Verification items for the finished model (mm, model axes). Round coordinates to 2 decimals unless told otherwise and drop trailing zeros. Write each loop counter-clockwise with the first axis right and the second up, starting at its lowest first coordinate (ties: lowest second). Pieces come first, ordered by that corner, then holes.
from build123d import *

# Parameters (mm, degrees)
GENERICCARDPCBDEFINITION_FILLET3_START   = -0.8
GENERICCARDPCBDEFINITION_FILLET3_OUTLI_R = 0.16
GENERICCARDPCBDEFINITION_FILLET3_DEPTH   = 1.6
SKETCH1_R                                = 1.1
CUT_EXTRUDE1_DEPTH                       = 10


# Read off the part's stored shape, not the designer's step: <GenericCardPCBDefinition>-<Fillet3>
with BuildPart() as part:
    # <GenericCardPCBDefinition>-<Fillet3> outli → <GenericCardPCBDefinition>-<Fillet3> (new body)
    with BuildSketch(Plane(origin=(0, 0, 0), x_dir=(1, 0, 0), z_dir=(0, 1, 0)).offset(GENERICCARDPCBDEFINITION_FILLET3_START)):
        with BuildLine():
            ThreePointArc((-41.232050808, -44.8), (-40.5, -44.067949192), (-39.5, -43.8))
            Line((-39.5, -43.8), (-38.267949192, -43.8))
            ThreePointArc((-38.267949192, -43.8), (-37.914395801, -43.653553391), (-37.767949192, -43.3))
            Line((-37.767949192, -43.3), (-37.767949192, -41.3))
            ThreePointArc((-37.767949192, -41.3), (-37.621502583, -40.946446609), (-37.267949192, -40.8))
            Line((-37.267949192, -40.8), (-35.59, -40.8))
            Line((-35.59, -40.8), (-35.59, -37.1))
            ThreePointArc((-35.59, -37.1), (-35.443553391, -36.746446609), (-35.09, -36.6))
            Line((-35.09, -36.6), (-32.91, -36.6))
            ThreePointArc((-32.91, -36.6), (-32.556446609, -36.746446609), (-32.41, -37.1))
            Line((-32.41, -37.1), (-32.41, -40.8))
            Line((-32.41, -40.8), (-29.59, -40.8))
            Line((-29.59, -40.8), (-29.59, -37.1))
            ThreePointArc((-29.59, -37.1), (-29.443553391, -36.746446609), (-29.09, -36.6))
            Line((-29.09, -36.6), (-26.91, -36.6))
            ThreePointArc((-26.91, -36.6), (-26.556446609, -36.746446609), (-26.41, -37.1))
            Line((-26.41, -37.1), (-26.41, -40.8))
            Line((-26.41, -40.8), (-23.59, -40.8))
            Line((-23.59, -40.8), (-23.59, -37.1))
            ThreePointArc((-23.59, -37.1), (-23.443553391, -36.746446609), (-23.09, -36.6))
            Line((-23.09, -36.6), (-20.91, -36.6))
            ThreePointArc((-20.91, -36.6), (-20.556446609, -36.746446609), (-20.41, -37.1))
            Line((-20.41, -37.1), (-20.41, -40.8))
            Line((-20.41, -40.8), (-18.732050808, -40.8))
            ThreePointArc((-18.732050808, -40.8), (-18.378497417, -40.946446609), (-18.232050808, -41.3))
            Line((-18.232050808, -41.3), (-18.232050808, -43.3))
            ThreePointArc((-18.232050808, -43.3), (-18.085604199, -43.653553391), (-17.732050808, -43.8))
            Line((-17.732050808, -43.8), (-16.5, -43.8))
            ThreePointArc((-16.5, -43.8), (-15.5, -44.067949192), (-14.767949192, -44.8))
            Line((-14.767949192, -44.8), (14.767949192, -44.8))
            ThreePointArc((14.767949192, -44.8), (16.5, -43.8), (18.232050808, -44.8))
            Line((18.232050808, -44.8), (37.767949192, -44.8))
            ThreePointArc((37.767949192, -44.8), (39.5, -43.8), (41.232050808, -44.8))
            Line((41.232050808, -44.8), (44.1, -44.8))
            Line((44.1, -44.8), (49.9, -39))
            Line((49.9, -39), (49.9, 40.9))
            ThreePointArc((49.9, 40.9), (49.753553391, 41.253553391), (49.4, 41.4))
            Line((49.4, 41.4), (47.65, 41.4))
            ThreePointArc((47.65, 41.4), (47.296446609, 41.546446609), (47.15, 41.9))
            Line((47.15, 41.9), (47.15, 45.8))
            ThreePointArc((47.15, 45.8), (47.003553391, 46.153553391), (46.65, 46.3))
            Line((46.65, 46.3), (34.9, 46.3))
            ThreePointArc((34.9, 46.3), (34.546446609, 46.446446609), (34.4, 46.8))
            Line((34.4, 46.8), (34.4, 49.4))
            ThreePointArc((34.4, 49.4), (34.253553391, 49.753553391), (33.9, 49.9))
            Line((33.9, 49.9), (-33.9, 49.9))
            ThreePointArc((-33.9, 49.9), (-34.253553391, 49.753553391), (-34.4, 49.4))
            Line((-34.4, 49.4), (-34.4, 46.8))
            ThreePointArc((-34.4, 46.8), (-34.546446609, 46.446446609), (-34.9, 46.3))
            Line((-34.9, 46.3), (-46.65, 46.3))
            ThreePointArc((-46.65, 46.3), (-47.003553391, 46.153553391), (-47.15, 45.8))
            Line((-47.15, 45.8), (-47.15, 41.9))
            ThreePointArc((-47.15, 41.9), (-47.296446609, 41.546446609), (-47.65, 41.4))
            Line((-47.65, 41.4), (-49.4, 41.4))
            ThreePointArc((-49.4, 41.4), (-49.753553391, 41.253553391), (-49.9, 40.9))
            Line((-49.9, 40.9), (-49.9, -39))
            Line((-49.9, -39), (-44.1, -44.8))
            Line((-44.1, -44.8), (-41.232050808, -44.8))
        make_face()
        with Locations((-35.59, -36.6)):
            Circle(GENERICCARDPCBDEFINITION_FILLET3_OUTLI_R, mode=Mode.SUBTRACT)
        with Locations((-32.41, -36.6)):
            Circle(GENERICCARDPCBDEFINITION_FILLET3_OUTLI_R, mode=Mode.SUBTRACT)
        with Locations((-29.59, -36.6)):
            Circle(GENERICCARDPCBDEFINITION_FILLET3_OUTLI_R, mode=Mode.SUBTRACT)
        with Locations((-26.41, -36.6)):
            Circle(GENERICCARDPCBDEFINITION_FILLET3_OUTLI_R, mode=Mode.SUBTRACT)
        with Locations((-23.59, -36.6)):
            Circle(GENERICCARDPCBDEFINITION_FILLET3_OUTLI_R, mode=Mode.SUBTRACT)
        with Locations((-20.41, -36.6)):
            Circle(GENERICCARDPCBDEFINITION_FILLET3_OUTLI_R, mode=Mode.SUBTRACT)
    extrude(amount=GENERICCARDPCBDEFINITION_FILLET3_DEPTH)

    # Sketch1 → Cut-Extrude1 (cut)
    with BuildSketch(Plane(origin=(0, 0.8, 0), x_dir=(1, 0, 0), z_dir=(0, 1, 0))):
        with Locations(Location((-17.3, -17.3, 0), (0, 0, 270))):
            Circle(SKETCH1_R)
        with Locations(Location((17.3, -17.3, 0), (0, 0, 270))):
            Circle(SKETCH1_R)
        with Locations(Location((-17.3, 17.3, 0), (0, 0, 270))):
            Circle(SKETCH1_R)
        with Locations(Location((17.3, 17.3, 0), (0, 0, 270))):
            Circle(SKETCH1_R)
        with BuildLine():
            Line((8.5, -8.5), (8.5, 8.5))
            Line((8.5, 8.5), (3, 8.5))
            Line((3, 8.5), (3, 9.5))
            ThreePointArc((3, 9.5), (0, 12.5), (-3, 9.5))
            Line((-3, 9.5), (-3, 8.5))
            Line((-3, 8.5), (-8.5, 8.5))
            Line((-8.5, 8.5), (-8.5, -8.5))
            Line((-8.5, -8.5), (-3, -8.5))
            Line((-3, -8.5), (-3, -9.5))
            ThreePointArc((-3, -9.5), (0, -12.5), (3, -9.5))
            Line((3, -9.5), (3, -8.5))
            Line((3, -8.5), (8.5, -8.5))
        make_face()
    extrude(amount=-CUT_EXTRUDE1_DEPTH, mode=Mode.SUBTRACT)


solid = part.part
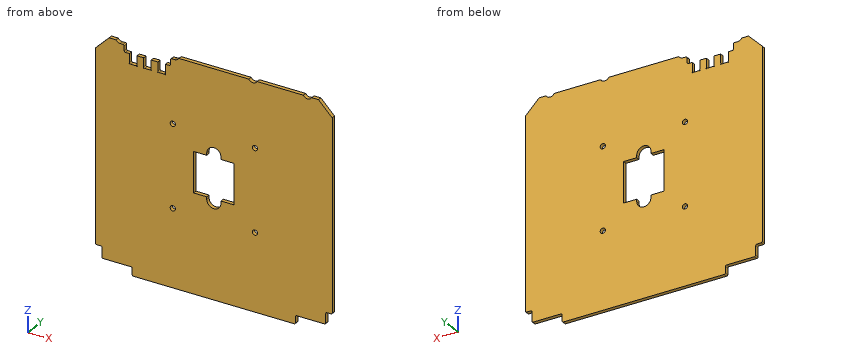
Q1. Depth check by flat-ended pin: P1, Ø0.5, axis at y = 0, z = -43, coming from the +X side; P2, Ø2, axis at x = -1.5, z = -10.5, coming from the +Y side; P3, Ø0.5, axis at x = -19, y = -0.5, coming from the +Z side; P4, Ø0.8, axis at x = -39.5, y = 0, coming from the -Z side. Enter the tip coordinate at first touch or a pass-through.
Recorded:
P1: stops at x = 47.15
P2: passes through
P3: stops at z = 40.8
P4: stops at z = -46.3
Q2. Sectioned sample at B-B (z = -6). Enter the section's corners in (x, y), plus the area to 3 significant figures.
Recorded:
outline: (-49.9, -0.8) - (-8.5, -0.8) - (-8.5, 0.8) - (-49.9, 0.8) - close; (8.5, -0.8) - (49.9, -0.8) - (49.9, 0.8) - (8.5, 0.8) - close
area: 132 mm2
Q3. Material ranges on line 1 along X through (y, z) = (-0.05, -17.3); line 2 along X through (y, z) = (0.35, -6.5); line 3 along Z through (x, y) = (43, -0.1), recorded low to high.
Recorded:
line 1: x = -49.9 to -18.4, -16.2 to 16.2, 18.4 to 49.9
line 2: x = -49.9 to -8.5, 8.5 to 49.9
line 3: z = -46.3 to 44.8
Q4. Sectioned sample at C-C (y = 0.3). Give the number of separate pieces and of enclosed holes in the cut face, plus the area to 3 significant figures.
Recorded:
separate pieces: 1
enclosed holes: 11
area: 8,810 mm2
Q5. Sectioned sample at A-A (x = 0). Enter the section's corners in (y, z), plus the area to 3 significant figures.
Recorded:
outline: (-0.8, -49.9) - (0.8, -49.9) - (0.8, -12.5) - (-0.8, -12.5) - close; (-0.8, 12.5) - (0.8, 12.5) - (0.8, 44.8) - (-0.8, 44.8) - close
area: 112 mm2
